CAD build for the part. Positions are in the model's coordinates, mm. Face numbers are marked on the shaded views. A direction names the side the tool comes from. Give positions to 0.01 mm unless a question says otherwise; leave off trailing zeros. Order: outer loops, then holes, each group sorted by start corner. A loop starts at its lowest first (then second) coordinate and runs counter-clockwise, first axis right, second up. Notation, with made-up numbers: M 18.5,-23.75 L 38.5,-23.75 A13 ccw 38.5,-5.75 Z; hole C -19.5,7.5 d8. An arc over 180 degrees is marked long. Put each result on its own line as item: value. Start each with the question number.
1) Tool access for the marked faces 4, 5 and 6: list every direction of +Z, -Z, +X, -X, +Y, -Y with a clear straight run to the whole face (end or side of a thin tool).
2) Cut at B-B (x = 5.3). Write the cut outline in (y, z).
3) Pin check, flat tips, straight feed: pin 1 (10 mm diameter, centred on x = 8, y = 19, fed in from -Z); pin 2 (5.5 mm diameter, centred on x = 3.5, y = 8, fed in from +Z); pin 3 (3 mm diameter, centred on x = 2, z = -1, fed in from +Y); pin 4 (3 mm diameter, centred on x = -4.5, y = 20.5, fed in from +Z). Stop position of each tip, or through.
4) Two-plate mould, pull along Z, no slides. Class the marked faces 1, 2 and 3: released by +Z, released by -Z, zero draft, split by the parting line, or undercut.
5) Cut at A-A (y = 9). Write the cut outline in (x, z).
6) Cut at C-C (z = 0). Write the cut outline in (x, y), and give its area (3 significant figures).
7) Drill centre lines: line 1 (Y direction, x = 5.3, z = -6.75); line 2 (X direction, y = 9, z = 9.15); line 3 (Z direction, x = 9.75, y = 14.25). Where is each one in solid material? Low to high. Write a range as [from, to].
8) Cut at D-D (y = 15.5). Write the cut outline in (x, z), and give its area (3 significant figures).
```python
from build123d import *

# Parameters (mm, degrees)
EXTRUDE_1_DEPTH     = 24.2
SHELL_1_T           = -1.7
EXTRUDE_2_REACH     = 38.885
SKETCH_2_R          = 8
SKETCH_2_R_2        = 6
SKETCH_3_R          = 4.5
CUT_EXTRUDE_1_DEPTH = 35.315157171
SKETCH_4_R          = 8
SKETCH_4_R_2        = 4.5
EXTRUDE_3_DEPTH     = 1


with BuildPart() as part:
    # 草圖1 → 填料-伸長1 (new body)
    with BuildSketch(Plane(origin=(0, 0, 0), x_dir=(1, 0, 0), z_dir=(0, 1, 0))):
        with BuildLine():
            Line((0, 7.9), (10.6, 7.9))
            ThreePointArc((10.6, 7.9), (18.5, 0), (10.6, -7.9))
            Line((10.6, -7.9), (0, -7.9))
            ThreePointArc((0, -7.9), (-7.9, 0), (0, 7.9))
        make_face()
    extrude(amount=EXTRUDE_1_DEPTH)

    # 薄殼1
    shell_1_openings = [part.faces().sort_by_distance(p)[0] for p in [
        (5.3, 24.2, 0),
    ]]
    offset(amount=SHELL_1_T, openings=shell_1_openings, kind=Kind.INTERSECTION)

    # 草圖2 → 填料-伸長2 (add, up to next)
    with BuildSketch(Plane.XY.offset(12.9), mode=Mode.PRIVATE) as extrude_2_sk1:
        with Locations((5.3, 9)):
            Circle(SKETCH_2_R)
        with Locations((5.3, 9)):
            Circle(SKETCH_2_R_2, mode=Mode.SUBTRACT)
    extrude_2_tool1 = extrude(extrude_2_sk1.sketch, amount=-EXTRUDE_2_REACH, mode=Mode.PRIVATE) - part.part
    add(extrude_2_tool1.solids().sort_by_distance((-2.473726, 9, 12.9))[0])

    # 草圖3 → 除料-伸長1 (cut, through all)
    with BuildSketch(Plane.XY.offset(7.9)):
        with Locations((5.3, 9)):
            Circle(SKETCH_3_R)
    extrude(amount=-CUT_EXTRUDE_1_DEPTH, mode=Mode.SUBTRACT)

    # 草圖4 → 填料-伸長3 (add)
    with BuildSketch(Plane(origin=(0, 0, -7.9), x_dir=(-1, 0, 0), z_dir=(0, 0, -1))):
        with Locations(Location((-5.3, 9, 0), (0, 0, 180))):
            Circle(SKETCH_4_R)
        with Locations(Location((-5.3, 9, 0), (0, 0, 180))):
            Circle(SKETCH_4_R_2, mode=Mode.SUBTRACT)
    extrude(amount=EXTRUDE_3_DEPTH)


solid = part.part
```
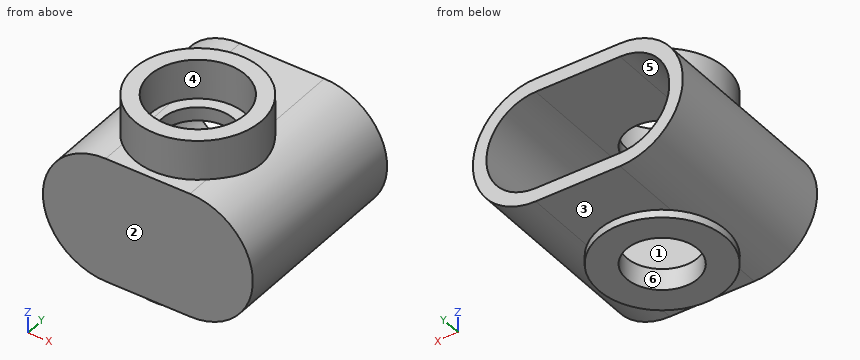
Solution:
1. face 4: +Z
1. face 5: +Y
1. face 6: +Z, -Z
2. outline: M 0,-7.9 L 1,-7.9 L 1,-8.9 L 4.5,-8.9 L 4.5,-6.2 L 1.7,-6.2 L 1.7,6.2 L 4.5,6.2 L 4.5,7.9 L 3,7.9 L 3,12.9 L 1,12.9 L 1,7.9 L 0,7.9 Z; M 13.5,-8.9 L 17,-8.9 L 17,-7.9 L 24.2,-7.9 L 24.2,-6.2 L 13.5,-6.2 Z; M 13.5,6.2 L 24.2,6.2 L 24.2,7.9 L 17,7.9 L 17,12.9 L 15,12.9 L 15,7.9 L 13.5,7.9 Z
3. pin 1: z = -8.9
3. pin 2: z = 7.9
3. pin 3: y = 1.7
3. pin 4: z = 7.31
4. face 1: undercut
4. face 2: zero draft
4. face 3: released by -Z
5. outline: M -2.7,-8.9 L 0.8,-8.9 L 0.8,-6.2 L 0,-6.2 A6.2 cw 0,6.2 L 0.8,6.2 L 0.8,7.9 L 0,7.9 A7.9 ccw -0.7,7.87 L -0.7,12.9 L -2.7,12.9 L -2.7,7.42 A7.9 ccw 0,-7.9 L -2.7,-7.9 Z; M 9.8,-8.9 L 13.3,-8.9 L 13.3,-7.9 L 10.6,-7.9 A7.9 ccw 13.3,7.42 L 13.3,12.9 L 11.3,12.9 L 11.3,7.87 A7.9 ccw 10.6,7.9 L 9.8,7.9 L 9.8,6.2 L 10.6,6.2 A6.2 cw 10.6,-6.2 L 9.8,-6.2 Z
6. outline: M -7.9,0 L 18.5,0 L 18.5,24.2 L 16.8,24.2 L 16.8,1.7 L -6.2,1.7 L -6.2,24.2 L -7.9,24.2 Z
6. area: 121 mm²
7. line 1: [0, 4.5], [13.5, 24.2]
7. line 2: [-2.7, -0.7], [11.3, 13.3]
7. line 3: [-8.9, -6.2], [6.2, 12.9]
8. outline: M 0,-7.9 L 0.64,-7.9 L 0.64,-8.9 L 9.96,-8.9 L 9.96,-7.9 L 10.6,-7.9 A7.9 ccw 10.6,7.9 L 9.96,7.9 L 9.96,12.9 L 0.64,12.9 L 0.64,7.9 L 0,7.9 A7.9 ccw Z; hole M 0,-6.2 L 10.6,-6.2 A6.2 ccw 10.6,6.2 L 0,6.2 A6.2 ccw Z
8. area: 167 mm²
